```python
from build123d import *

# Parameters (mm, degrees)
F0_W      = 76.2886032462
F0_H      = 151.6468524933
F1_DEPTH  = 76.454
F2_T      = -2.54
F3_W      = 71.2086032462
F3_H      = 2.0932815969
F4_DEPTH  = 73.914
F5_W      = 3.2325349748
F5_H      = 127.0110753989
F6_DEPTH  = 73.66
F7_W      = 32.3717666483
F7_H      = 2.0932848565
F8_DEPTH  = 73.66
F10_W     = 35.353255691
F10_H     = 2.0932848565
F11_DEPTH = 73.66
F9_W      = 35.6043016231
F9_H      = 2.7910489589
F12_DEPTH = 73.66
F16_W     = 25.3520011902
F16_H     = 3.7214010954
F17_DEPTH = 49.784
F15_W     = 3.0236318707
F15_H     = 68.8458192162
F18_DEPTH = 50.292
F14_W     = 28.8408100605
F14_H     = 1.6281104181
F19_DEPTH = 50.546
F13_W     = 2.9977930403
F13_H     = 71.1901413901
F20_DEPTH = 50.292
F22_DEPTH = 47.498
F23_DEPTH = 73.406


with BuildPart() as f1:
    # F0 (on Front) → F1 (new body)
    with BuildSketch(Plane.XZ):
        with Locations((-38.1443016231, 0)):
            Rectangle(F0_W, F0_H)
    extrude(amount=-F1_DEPTH)

    # F2
    f2_openings = [f1.faces().sort_by_distance(p)[0] for p in [
        (-38.144302, 0, 0),
    ]]
    offset(amount=F2_T, openings=f2_openings)

    # F3 (on face) → F4 (join)
    with BuildSketch(Plane.XZ.offset(-73.914)):
        with Locations((-38.1443016231, 54.7742899507)):
            Rectangle(F3_W, F3_H)
    extrude(amount=F4_DEPTH)

    # F5 (on face) → F6 (join)
    with BuildSketch(Plane.XZ.offset(-73.914)):
        with Locations((-39.7605691105, -9.7778885472)):
            Rectangle(F5_W, F5_H)
    extrude(amount=F6_DEPTH)

    # F7 (on face) → F8 (join)
    with BuildSketch(Plane.XZ.offset(-73.914)):
        with Locations((-57.5627199221, -1.0466424283)):
            Rectangle(F7_W, F7_H)
    extrude(amount=F8_DEPTH)

    # F10 (on face) → F11 (join)
    with BuildSketch(Plane.XZ.offset(-73.914)):
        with Locations((-20.0468016556, -1.0466424283)):
            Rectangle(F10_W, F10_H)
    extrude(amount=F11_DEPTH)

    # F9 (on face) → F12 (join)
    with BuildSketch(Plane.XZ.offset(-73.914)):
        with Locations((-20.3421508116, 29.7711631283)):
            Rectangle(F9_W, F9_H)
    extrude(amount=F12_DEPTH)

    # F16 (on face) → F17 (join)
    with BuildSketch(Plane.XZ.offset(-73.914)):
        with Locations((-58.0748096108, -71.1716860533)):
            Rectangle(F16_W, F16_H)
    extrude(amount=-F17_DEPTH)

    # F15 (on face) → F18 (join)
    with BuildSketch(Plane.XZ.offset(-73.914)):
        with Locations((-43.4218160808, -38.3768922184)):
            Rectangle(F15_W, F15_H)
    extrude(amount=-F18_DEPTH)

    # F14 (on face) → F19 (join)
    with BuildSketch(Plane.XZ.offset(-73.914)):
        with Locations((-56.3304051757, -3.372514504)):
            Rectangle(F14_W, F14_H)
    extrude(amount=-F19_DEPTH)

    # F13 (on face) → F20 (join)
    with BuildSketch(Plane.XZ.offset(-73.914)):
        with Locations((-72.2497067261, -37.6883555516)):
            Rectangle(F13_W, F13_H)
    extrude(amount=-F20_DEPTH)

    # F21 (on face) → F22 (join)
    with BuildSketch(Plane(origin=(0, 76.454, 0), x_dir=(-1, 0, 0), z_dir=(0, 1, 0))):
        Polygon((70.7508102059, -4.1865697131), (44.9336320162, -4.1865697131), (44.9336320162, -69.3109855056), (45.3988090158, -69.3109855056), (70.7508102059, -69.3109855056), align=None)
    extrude(amount=F22_DEPTH)

    # F23 (add): a face of the model
    f23_faces = [f1.faces().sort_by_distance(p)[0] for p in [
        (-57.5627199221, 73.914, -37.6883555516),
    ]]
    extrude(f23_faces, amount=F23_DEPTH)


solid = f1.part
```
CAD build for the part. Positions are in the model's coordinates, mm. A direction names the side the tool comes from. Coordinates: 2 decimals unless noted, no trailing zeros. Write each loop counter-clockwise with the first axis right and the second up, starting at its lowest first coordinate (ties: lowest second). Pieces come first, ordered by that corner, then holes.
(1) Drill centre lines: probe 1 along X at (y, z) = (29, 1.5); probe 2 along Z at (x, y) = (-60, 29); probe 3 along Z at (x, y) = (-21, 57.5). Where is each one in solid material? Low to high.
(2) Flat gauge pins, fed straight in: pin 1 (2 mm diameter, centred on x = -20.5, z = -24.5, fed in from -Y); pin 2 (1.5 mm diameter, centred on x = -65.5, y = 81.5, fed in from -Z); pin 3 (1 mm diameter, centred on x = -35.5, z = -4, fed in from +Y). Where does each tip first touch, or does it go through?
(3) Cut at A-A, the plane z = -45.5. List the corners of the cut face in (x, y), and give its area (3 significant figures).
(4) Cut at D-D, the plane y = 97.5. List the corners of the cut face in (x, z), and give its area (3 significant figures).
(5) 3-axis set-ups, long thin cutter, end or side, ignore diameter. For faces 4 (the face through (-58, 123.698, -71)), 5 (the face through (-21, 38, 28.376)): which of +Z, -Z, +X, -X, +Y, -Y reach the whole face in a straight line?
(6) Cut at B-B, the plane x = -5. List the corners of the cut face in (y, z).
(7) Two-plate mould, pull along X, no slides. Class faces 1 (the face through (-39, 38, 75.823)), 2 (the face through (-73.749, 100, -38)), 3 (the face through (-20, 38, 0)): +X half, -X half, draft (parallel to the pull), parting line (faces both ways), or undercut.
(8) Cut at C-C, the plane y = 42. List the corners of the cut face in (x, z), and give its area (3 significant figures).
Geometry says:
1. probe 1: x = -76.29 to -73.75, -41.38 to -38.14, -2.54 to 0
1. probe 2: z = -75.82 to 0, 53.73 to 55.82, 73.28 to 75.82
1. probe 3: z = -75.82 to -73.28, -2.09 to 0, 28.38 to 31.17, 53.73 to 55.82, 73.28 to 75.82
2. pin 1: stops at y = 73.91
2. pin 2: stops at z = -73.03
2. pin 3: stops at y = 76.45
3. outline: (-76.29, 0) - (-73.75, 0) - (-73.75, 0.51) - (-41.38, 0.51) - (-41.38, 0.25) - (-38.14, 0.25) - (-38.14, 73.91) - (-2.54, 73.91) - (-2.54, 0) - (0, 0) - (0, 76.45) - (-41.91, 76.45) - (-41.91, 124.21) - (-44.93, 124.21) - (-44.93, 123.95) - (-70.75, 123.95) - (-70.75, 124.21) - (-73.75, 124.21) - (-73.75, 76.45) - (-76.29, 76.45) - close
3. area: 4,700 mm2
4. outline: (-73.75, -73.28) - (-70.75, -73.28) - (-70.75, -73.03) - (-45.4, -73.03) - (-45.4, -69.31) - (-44.93, -69.31) - (-44.93, -72.8) - (-41.91, -72.8) - (-41.91, -2.56) - (-70.75, -2.56) - (-70.75, -2.09) - (-73.75, -2.09) - close
4. area: 2,240 mm2
5. face 4: -Z, +Y
5. face 5: -Y
6. outline: (0, -75.82) - (76.45, -75.82) - (76.45, 75.82) - (0, 75.82) - (0, 73.28) - (73.91, 73.28) - (73.91, 55.82) - (0, 55.82) - (0, 53.73) - (73.91, 53.73) - (73.91, 31.17) - (0.25, 31.17) - (0.25, 28.38) - (73.91, 28.38) - (73.91, 0) - (0.25, 0) - (0.25, -2.09) - (73.91, -2.09) - (73.91, -73.28) - (0, -73.28) - close
7. face 1: draft
7. face 2: -X half
7. face 3: undercut
8. outline: (-76.29, -75.82) - (0, -75.82) - (0, 75.82) - (-76.29, 75.82) - close; hole (-73.75, 0) - (-41.38, 0) - (-41.38, 53.73) - (-73.75, 53.73) - close; hole (-73.75, 55.82) - (-2.54, 55.82) - (-2.54, 73.28) - (-73.75, 73.28) - close; hole (-38.14, -73.28) - (-2.54, -73.28) - (-2.54, -2.09) - (-37.72, -2.09) - (-37.72, 0) - (-2.54, 0) - (-2.54, 28.38) - (-38.14, 28.38) - close; hole (-38.14, 31.17) - (-2.54, 31.17) - (-2.54, 53.73) - (-38.14, 53.73) - close
8. area: 4,240 mm2
